The model under review builds one solid part; all positions refer to its coordinate system, in mm. A direction names the side the tool comes from. Round coordinates to 2 decimals unless told otherwise and drop trailing zeros. Loops run counter-clockwise (first coordinate to the right, second up) from the corner with the lowest first, then second, coordinate; pieces in that order, holes last. Notation, with made-up numbers: M -6.5,31 L -2.5,31 A19 ccw -2.5,50 Z; hole C -14,-7.5 d5. An arc over 180 degrees is marked long. Return JSON: item names as keys, results as strings. Group by question number.
Q1. Consider section B-B (z = 14). State the section outline as (x, y) points (3 decimals), and give its area (3 significant figures).
Q2. Consider section A-A (y = -17.25). State the section outline as (x, z) points.
Q3. Draft analysis for pull direction Z (two halves, no side actions). For faces 1 (the face through (30, -24, 0)), 2 (the face through (39.286, -25.531, 13.68)), 3 (the face through (25.04, -16.38, 10.11)), 4 (the face through (39, -27.096, 15)), state which applies: pulls with the +Z half, pulls with the -Z half, needs draft (parallel to the pull), parting line crosses it, or undercut.
Q4. Clearance check with flat-ended pins moving along their axes: pin 1 Ø12 at (x, z) = (35, 20) entering from +Y; pin 2 Ø5 at (y, z) = (-14.5, 9.5) entering from -X. State where each tip first meets the part, or that it passes through.
Q5. For faces 5 (the face through (40, -23.921, 13)), 6 (the face through (23.473, -17, 15)), list the 3-axis set-ups (+Z, -Z, +X, -X, +Y, -Y) from which the entire face can be reached by the end or side of a thin tool; tool diameter is ignored.
Q6. Consider section C-C (x = 43.75). State the section outline as (y, z) points, and give its area (3 significant figures).
Q7. To check wall thickness, follow line 1 along Y through (x, z) = (36.25, 1.5); line 2 along X through (y, z) = (-10.75, 19.75); line 3 along Y through (x, z) = (25.9, 12.7). State the ranges of each line that lie inside material, in increasing order.
Q8. Consider section D-D (y = -12). State the section outline as (x, z) points, and give its area (3 significant figures).
from build123d import *

# Parameters (mm, degrees)
EXTRUDE1_DEPTH     = 25.4
SKETCH2_R          = 3.2639
CUT_EXTRUDE1_DEPTH = 26.4
SKETCH3_R          = 3.2639
CUT_EXTRUDE2_DEPTH = 26.4


with BuildPart() as part:
    # Sketch1 → Extrude1 (new body)
    with BuildSketch(Plane.XY):
        with BuildLine():
            Line((23.473046964, -1.696403207), (23.473046964, -27.096403207))
            Line((23.473046964, -27.096403207), (48.873046964, -27.096403207))
            ThreePointArc((48.873046964, -27.096403207), (47.943110995, -24.851339177), (45.698046964, -23.921403207))
            Line((45.698046964, -23.921403207), (31.423246964, -23.921403207))
            ThreePointArc((31.423246964, -23.921403207), (28.046670663, -22.522779509), (26.648046964, -19.146203207))
            Line((26.648046964, -19.146203207), (26.648046964, -4.871403207))
            ThreePointArc((26.648046964, -4.871403207), (25.718110995, -2.626339177), (23.473046964, -1.696403207))
        make_face()
    extrude(amount=EXTRUDE1_DEPTH)

    # Sketch2 → Cut-Extrude1 (cut, through all)
    with BuildSketch(Plane.ZY.offset(-23.473046964)):
        with Locations((12.7, -14.396403207)):
            Circle(SKETCH2_R)
    extrude(amount=-CUT_EXTRUDE1_DEPTH, mode=Mode.SUBTRACT)

    # Sketch3 → Cut-Extrude2 (cut, through all)
    with BuildSketch(Plane.XZ.offset(27.096403207)):
        with Locations((36.173046964, 12.7)):
            Circle(SKETCH3_R)
    extrude(amount=-CUT_EXTRUDE2_DEPTH, mode=Mode.SUBTRACT)


solid = part.part
Values:
{
 "1": {"outline": "M 23.473,-27.096 L 33.179,-27.096 L 33.179,-23.921 L 31.423,-23.921 A4.775 cw 26.648,-19.146 L 26.648,-17.39 L 23.473,-17.39 Z; M 23.473,-11.403 L 26.648,-11.403 L 26.648,-4.871 A3.175 ccw 23.473,-1.696 Z; M 39.167,-27.096 L 48.873,-27.096 A3.175 ccw 45.698,-23.921 L 39.167,-23.921 Z", "area": "114 mm2"},
 "2": {"outline": "M 23.47,0 L 26.65,0 L 26.65,11.12 L 23.47,11.12 Z; M 23.47,14.28 L 26.65,14.28 L 26.65,25.4 L 23.47,25.4 Z"},
 "3": {"face 1": "pulls with the -Z half", "face 2": "undercut", "face 3": "undercut", "face 4": "needs draft"},
 "4": {"pin 1": "stops at y = -23.26", "pin 2": "stops at x = 23.47"},
 "5": {"face 5": "+Z, -Z, +X, +Y", "face 6": "+Z, -Z, -X, +Y, -Y"},
 "6": {"outline": "M -27.1,0 L -23.92,0 L -23.92,25.4 L -27.1,25.4 Z", "area": "80.6 mm2"},
 "7": {"line 1": "y = -27.1 to -23.92", "line 2": "x = 23.47 to 26.65", "line 3": "y = -27.1 to -17.66, -11.13 to -2.82"},
 "8": {"outline": "M 23.47,0 L 26.65,0 L 26.65,10.48 L 23.47,10.48 Z; M 23.47,14.92 L 26.65,14.92 L 26.65,25.4 L 23.47,25.4 Z", "area": "66.6 mm2"}
}
